Input: part model. Units: mm. Frame: model coordinates. Face numbers are marked on the shaded views. A direction names the side the tool comes from. Coordinates: 2 decimals unless noted, no trailing zeros. Loops run counter-clockwise (first coordinate to the right, second up) from the corner with the lowest first, then second, coordinate; pieces in that order, holes last. Notation, with made-up numbers: (58.25, 2) - (77.25, 2) arc R13 cw to (77.25, 13) - close; hole circle Ø3 at (72.25, -32). An arc over 180 degrees is marked (long way). Use one line per item in the form item = value.
from build123d import *

# Parameters (mm, degrees)
ESBO_O1_W                                           = 74
ESBO_O1_H                                           = 74
RESSALTO_EXTRUS_O1_DEPTH                            = 25
CHANFRO1_SIZE                                       = 1.5
REBAIXO_PARA_PARAFUSO_COM_CABE_A_PANELA_D           = 50
REBAIXO_PARA_PARAFUSO_COM_CABE_A_PANELA_DEPTH       = 35
REBAIXO_PARA_PARAFUSO_COM_CABE_A_PANELA_CBORE_D     = 66
REBAIXO_PARA_PARAFUSO_COM_CABE_A_PANELA_CBORE_DEPTH = 3
REBAIXO_PARA_PARAFUSO_COM_CABE_A_PANELA_TIP         = 15.021515476
ESBO_O4_W                                           = 10
ESBO_O4_H                                           = 50
CORTE_EXTRUS_O1_DEPTH                               = 16.4
ESBO_O6_W                                           = 10
ESBO_O6_H                                           = 50
CORTE_EXTRUS_O2_DEPTH                               = 16.4
CORTE_EXTRUS_O4_REACH                               = 19.461
ESBO_O11_W                                          = 10
ESBO_O11_H                                          = 50
CORTE_EXTRUS_O3_DEPTH                               = 7
PADR_OCIRCULAR1_COUNT                               = 4
ESBO_O13_R                                          = 33
ESBO_O13_R_2                                        = 25
RESSALTO_EXTRUS_O2_DEPTH                            = 2
ESBO_O14_R                                          = 35.5
ESBO_O14_R_2                                        = 33
CORTE_EXTRUS_O5_DEPTH                               = 3.5
CORTE_EXTRUS_O10_DEPTH                              = 8
PADR_OCIRCULAR2_COUNT                               = 4
FILETE1_R                                           = 0.25
FILETE2_R                                           = 0.15


with BuildPart() as part:
    # Esboço1 → Ressalto-extrusão1 (new body)
    with BuildSketch(Plane(origin=(0, 0, 0), x_dir=(0, 0, -1), z_dir=(1, 0, 0))):
        with Locations((37, 37)):
            Rectangle(ESBO_O1_W, ESBO_O1_H)
    extrude(amount=RESSALTO_EXTRUS_O1_DEPTH)

    # Chanfro1
    chanfro1_edges = [part.edges().sort_by_distance(p)[0] for p in [
        (12.5, 74, 0),
        (12.5, 74, -74),
        (12.5, 0, -74),
        (12.5, 0, 0),
    ]]
    chamfer(chanfro1_edges, length=CHANFRO1_SIZE)

    # Rebaixo para parafuso com cabeça panela de M21
    with Locations(Plane(origin=(25, 0, 0), x_dir=(0, 0, -1), z_dir=(1, 0, 0))):
        with Locations((37, 37)):
            CounterBoreHole(REBAIXO_PARA_PARAFUSO_COM_CABE_A_PANELA_D / 2, REBAIXO_PARA_PARAFUSO_COM_CABE_A_PANELA_CBORE_D / 2, REBAIXO_PARA_PARAFUSO_COM_CABE_A_PANELA_CBORE_DEPTH, depth=REBAIXO_PARA_PARAFUSO_COM_CABE_A_PANELA_DEPTH)
            with Locations((0, 0, -(REBAIXO_PARA_PARAFUSO_COM_CABE_A_PANELA_DEPTH + REBAIXO_PARA_PARAFUSO_COM_CABE_A_PANELA_TIP / 2))):  # 118° drill point
                Cone(0, REBAIXO_PARA_PARAFUSO_COM_CABE_A_PANELA_D / 2, REBAIXO_PARA_PARAFUSO_COM_CABE_A_PANELA_TIP, mode=Mode.SUBTRACT)

    # Esboço4 → Corte-extrusão1 (cut)
    with BuildSketch(Plane(origin=(0, 12.346551211, -12.346551211), x_dir=(1, 0, 0), z_dir=(0, -0.707106781, 0.707106781))):
        with Locations((13, 0)):
            Rectangle(ESBO_O4_W, ESBO_O4_H)
    corte_extrus_o1 = extrude(amount=CORTE_EXTRUS_O1_DEPTH, mode=Mode.SUBTRACT)

    # Espelhar1: Corte-extrusão1 across plane
    add(corte_extrus_o1.mirror(Plane(origin=(0, 37, -37), x_dir=(0, 0.707106781, 0.707106781), z_dir=(0, -0.707106781, 0.707106781))), mode=Mode.SUBTRACT)

    # Esboço6 → Corte-extrusão2 (cut)
    with BuildSketch(Plane(origin=(0, -36.25, -36.25), x_dir=(1, 0, 0), z_dir=(0, -0.707106781, -0.707106781))):
        with Locations((13, -52.325901808)):
            Rectangle(ESBO_O6_W, ESBO_O6_H)
    extrude(amount=-CORTE_EXTRUS_O2_DEPTH, mode=Mode.SUBTRACT)

    # Esboço11 → Corte-extrusão4 (cut, up to next)
    with BuildSketch(Plane(origin=(0, 24.653448789, 24.653448789), x_dir=(1, 0, 0), z_dir=(0, 0.707106781, 0.707106781)), mode=Mode.PRIVATE) as corte_extrus_o4_sk1:
        with Locations((13, 52.325901808)):
            Rectangle(ESBO_O11_W, ESBO_O11_H)
    corte_extrus_o4_tool1 = extrude(corte_extrus_o4_sk1.sketch, amount=CORTE_EXTRUS_O4_REACH, mode=Mode.PRIVATE) & part.part
    add(corte_extrus_o4_tool1.solids().sort_by_distance((13, 61.653449, -12.346551))[0], mode=Mode.SUBTRACT)

    # Esboço9 → Corte-extrusão3 (cut)
    with BuildSketch(Plane(origin=(25, 0, 0), x_dir=(0, 0, -1), z_dir=(1, 0, 0))):
        with BuildLine():
            Line((8.110912703, 74), (4.055456352, 69.944543648))
            ThreePointArc((4.055456352, 69.944543648), (3.852112704, 66.282711392), (7.468916653, 65.675180896))
            ThreePointArc((7.468916653, 65.675180896), (7.630037959, 65.785169024), (7.782956276, 65.90630305))
            ThreePointArc((7.782956276, 65.90630305), (7.937911293, 66.062088707), (8.09369695, 66.217043724))
            ThreePointArc((8.09369695, 66.217043724), (13.278272682, 70.563218753), (19.105587464, 74))
            Line((19.105587464, 74), (8.110912703, 74))
        make_face()
    corte_extrus_o3 = extrude(amount=-CORTE_EXTRUS_O3_DEPTH, mode=Mode.SUBTRACT)

    # PadrãoCircular1: Corte-extrusão3 ×4 about axis
    padr_ocircular1_axis = Axis((0, 37, -37), (1, 0, 0))
    for i in range(1, PADR_OCIRCULAR1_COUNT):
        add(corte_extrus_o3.rotate(padr_ocircular1_axis, i * 360 / PADR_OCIRCULAR1_COUNT), mode=Mode.SUBTRACT)

    # Esboço13 → Ressalto-extrusão2 (add)
    with BuildSketch(Plane.ZY):
        with Locations((-37, 37)):
            Circle(ESBO_O13_R)
        with Locations((-37, 37)):
            Circle(ESBO_O13_R_2, mode=Mode.SUBTRACT)
    extrude(amount=RESSALTO_EXTRUS_O2_DEPTH)

    # Esboço14 → Corte-extrusão5 (cut)
    with BuildSketch(Plane.ZY.offset(2)):
        with Locations((-37, 37)):
            Circle(ESBO_O14_R)
        with Locations((-37, 37)):
            Circle(ESBO_O14_R_2, mode=Mode.SUBTRACT)
    extrude(amount=-CORTE_EXTRUS_O5_DEPTH, mode=Mode.SUBTRACT)

    # Esboço16 → Corte-extrusão10 (cut)
    with BuildSketch(Plane.ZY):
        with BuildLine():
            ThreePointArc((-7.782956276, 65.90630305), (-3.979263896, 66.134758569), (-4.055456352, 69.944543648))
            Line((-4.055456352, 69.944543648), (-8.110912703, 74))
            Line((-8.110912703, 74), (-19.105587464, 74))
            ThreePointArc((-19.105587464, 74), (-13.278272682, 70.563218753), (-8.09369695, 66.217043724))
            ThreePointArc((-8.09369695, 66.217043724), (-7.937911293, 66.062088707), (-7.782956276, 65.90630305))
        make_face()
    corte_extrus_o10 = extrude(amount=-CORTE_EXTRUS_O10_DEPTH, mode=Mode.SUBTRACT)

    # PadrãoCircular2: Corte-extrusão10 ×4 about axis
    padr_ocircular2_axis = Axis((0, 37, -37), (1, 0, 0))
    for i in range(1, PADR_OCIRCULAR2_COUNT):
        add(corte_extrus_o10.rotate(padr_ocircular2_axis, i * 360 / PADR_OCIRCULAR2_COUNT), mode=Mode.SUBTRACT)

    # Filete1
    filete1_edges = [part.edges().sort_by_distance(p)[0] for p in [
        (1.5, 37, -72.5),
        (1.5, 37, -70),
    ]]
    fillet(filete1_edges, radius=FILETE1_R)

    # Filete2
    filete2_edges = [part.edges().sort_by_distance(p)[0] for p in [
        (0, 37, -72.5),
    ]]
    fillet(filete2_edges, radius=FILETE2_R)


solid = part.part
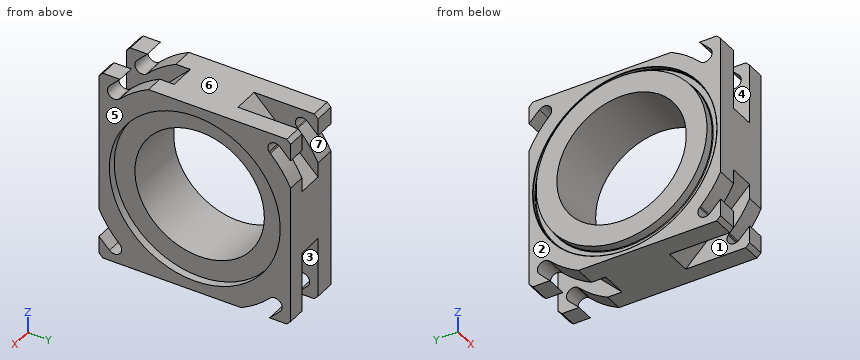
Q1. Cut plane D-D, the plane x = 10.25. Return loops of the section in (y, z).
Check values:
outline = (0, -49.31) - (24.69, -74) - (49.31, -74) - (74, -49.31) - (74, -24.69) - (49.31, 0) - (24.69, 0) - (0, -24.69) - close; hole circle Ø50 at (37, -37)
Q2. First-contact query: P1, Ø20, axis at y = 52, z = -52.5, coming from the +X side. Flat tip, straight axial feed; report the tip coordinate or a pass-through.
Check values:
P1 = 22
Q3. Cut plane C-C, the plane y = 37. Return loops of the section in (x, z), then the cut area to 3 significant figures.
Check values:
outline = (-2, -70) - (1.25, -70) arc R0.25 cw to (1.5, -70.25) - (1.5, -72.25) arc R0.25 cw to (1.25, -72.5) - (0.15, -72.5) arc R0.15 ccw to (0, -72.65) - (0, -74) - (25, -74) - (25, -70) - (22, -70) - (22, -62) - (-2, -62) - close; (-2, -12) - (22, -12) - (22, -4) - (25, -4) - (25, 0) - (0, 0) - (0, -1.35) arc R0.15 ccw to (0.15, -1.5) - (1.25, -1.5) arc R0.25 cw to (1.5, -1.75) - (1.5, -3.75) arc R0.25 cw to (1.25, -4) - (-2, -4) - close
area = 577 mm²
Q4. Set-up query: the marked faces 1, 2, 3 and 4. Return all of +Z, -Z, +X, -X, +Y, -Y with unobstructed straight access to the full face (end or side cutting, diameter ignored); none if empty.
Check values:
face_1 = -Z, -Y
face_2 = -X
face_3 = -Z, +Y
face_4 = +Z, -Y
Q5. Cut plane A-A, the plane z = -37. Return loops of the section in (x, y).
Check values:
outline = (-2, 4) - (1.25, 4) arc R0.25 cw to (1.5, 3.75) - (1.5, 1.75) arc R0.25 cw to (1.25, 1.5) - (0.15, 1.5) arc R0.15 ccw to (0, 1.35) - (0, 0) - (25, 0) - (25, 4) - (22, 4) - (22, 12) - (-2, 12) - close; (-2, 62) - (22, 62) - (22, 70) - (25, 70) - (25, 74) - (0, 74) - (0, 72.65) arc R0.15 ccw to (0.15, 72.5) - (1.25, 72.5) arc R0.25 cw to (1.5, 72.25) - (1.5, 70.25) arc R0.25 cw to (1.25, 70) - (-2, 70) - close
Q6. Ray query, line 1 along Y through (x, z) = (1, -37); line 2 along X through (y, z) = (57.5, -6); line 3 along Y through (x, z) = (3, -7). Return the intervals inside material, ascending. Write a range as [from, to].
Check values:
line_1 = [0, 1.5], [4, 12], [62, 70], [72.5, 74]
line_2 = [0, 8], [18, 25]
line_3 = [0, 3.44], [8.91, 65.44], [72.89, 74]
Q7. Pull-direction query (Z, two-part tool) for the marked faces 5, 6 and 7; classes: pulls with the +Z half, pulls with the -Z half, needs draft (parallel to the pull), parting line crosses it, or undercut.
Check values:
face_5 = needs draft
face_6 = pulls with the +Z half
face_7 = undercut
